from build123d import *


with BuildPart() as part:
    # Esquisse1 → Révolution1 (revolve)
    with BuildSketch(Plane.XY, mode=Mode.PRIVATE) as r_volution1_sk:
        with BuildLine():
            Line((7, 51.583866339), (7, 47.083866339))
            Line((7, 47.083866339), (9.414213562, 47.083866339))
            ThreePointArc((9.414213562, 47.083866339), (9.796896995, 47.007745871), (10.121320344, 46.79097312))
            Line((10.121320344, 46.79097312), (12.414213562, 44.498079901))
            ThreePointArc((12.414213562, 44.498079901), (12.847759065, 43.849233203), (13, 43.083866339))
            Line((13, 43.083866339), (13, 38.583866339))
            Line((13, 38.583866339), (12, 38.583866339))
            Line((12, 38.583866339), (12, 43.083866339))
            ThreePointArc((12, 43.083866339), (11.923879533, 43.466549771), (11.707106781, 43.79097312))
            Line((11.707106781, 43.79097312), (9.414213562, 46.083866339))
            Line((9.414213562, 46.083866339), (7, 46.083866339))
            ThreePointArc((7, 46.083866339), (6.292893219, 46.376759557), (6, 47.083866339))
            Line((6, 47.083866339), (6, 51.583866339))
            Line((6, 51.583866339), (7, 51.583866339))
        make_face()
    revolve(r_volution1_sk.sketch.rotate(Axis((0, 0, 0), (0, 1, 0)), 90), axis=Axis((0, 0, 0), (0, 1, 0)))


solid = part.part
Model file for the job. Use its own axes, mm. A direction names the side the tool comes from. Coordinates: 2 decimals unless noted, no trailing zeros. Order: outer loops, then holes, each group sorted by start corner. A loop starts at its lowest first (then second) coordinate and runs counter-clockwise, first axis right, second up. Notation, with made-up numbers: M -33.5,45 L -16.5,45 A19 ccw -16.5,72 Z; hole C 65,53.5 d8. An arc over 180 degrees is marked long. Return JSON: item names as keys, results as strings.
1. Tool access for faces 4 (the face through (-3.604, 40.865, -11.446)), 5 (the face through (6.21, 49.3, -3.23)), 6 (the face through (-2, 51.584, 6)): list every direction of +Z, -Z, +X, -X, +Y, -Y with a clear straight run to the whole face (end or side of a thin tool).
Ans:
{"face 4": "-Y", "face 5": "+Y", "face 6": "+Z, -Z, +X, -X, +Y"}
2. Saw through at B-B (x = 0). Give the cut face in (y, z).
Ans:
{"outline": "M 38.58,-13 L 43.08,-13 A2 ccw 44.5,-12.41 L 46.79,-10.12 A1 ccw 47.08,-9.41 L 47.08,-7 L 51.58,-7 L 51.58,-6 L 47.08,-6 A1 ccw 46.08,-7 L 46.08,-9.41 L 43.79,-11.71 A1 cw 43.08,-12 L 38.58,-12 Z; M 38.58,12 L 43.08,12 A1 cw 43.79,11.71 L 46.08,9.41 L 46.08,7 A1 ccw 47.08,6 L 51.58,6 L 51.58,7 L 47.08,7 L 47.08,9.41 A1 ccw 46.79,10.12 L 44.5,12.41 A2 ccw 43.08,13 L 38.58,13 Z"}
3. Pull direction X, two halves, no side cores. Call faces 1 (the face through (-7.02, 47.084, -1.44)), 2 (the face through (7.91, 40.802, 10.316)), 3 (the face through (-1.802, 49.365, -5.723)): +X half, -X half, draft (parallel to the pull), parting line (faces both ways), or undercut.
Ans:
{"face 1": "draft", "face 2": "parting line", "face 3": "undercut"}
4. Drill centre lines: probe 1 along X at (y, z) = (40.35, 0); probe 2 along X at (y, z) = (49.7, 0); probe 3 along Z at (x, y) = (9.5, 41). Where is each one in solid material? Low to high.
Ans:
{"probe 1": "-13 to -12, 12 to 13", "probe 2": "-7 to -6, 6 to 7", "probe 3": "-8.87 to -7.33, 7.33 to 8.87"}
5. Saw through at C-C (y = 41). Give the cut face in (x, z).
Ans:
{"outline": "C 0,0 d26; hole C 0,0 d24"}
6. Flat gauge pins, fed straight in: pin 1 (3 mm diameter, centred on y = 44, z = -9, fed in from +X); pin 2 (3 mm diameter, centred on x = -9.5, y = 42.5, fed in from +Z); pin 3 (1.5 mm diameter, centred on y = 41, z = 3, fed in from -X); pin 4 (6 mm diameter, centred on x = -2, y = 44.5, fed in from -Z). Where does each tip first touch, or does it go through?
Ans:
{"pin 1": "x = 10.5", "pin 2": "z = 10.25", "pin 3": "x = -12.8", "pin 4": "z = -13"}
7. Saw through at A-A (z = 0). Give the cut face in (x, y).
Ans:
{"outline": "M -13,38.58 L -12,38.58 L -12,43.08 A1 cw -11.71,43.79 L -9.41,46.08 L -7,46.08 A1 ccw -6,47.08 L -6,51.58 L -7,51.58 L -7,47.08 L -9.41,47.08 A1 ccw -10.12,46.79 L -12.41,44.5 A2 ccw -13,43.08 Z; M 6,47.08 A1 ccw 7,46.08 L 9.41,46.08 L 11.71,43.79 A1 cw 12,43.08 L 12,38.58 L 13,38.58 L 13,43.08 A2 ccw 12.41,44.5 L 10.12,46.79 A1 ccw 9.41,47.08 L 7,47.08 L 7,51.58 L 6,51.58 Z"}
